Can you work these out from the model? Positions are in its coordinate system, mm. Round coordinates to 2 decimals unless told otherwise and drop trailing zeros. Order: outer loops, then holes, each group sorted by start corner. A loop starts at its lowest first (then second) coordinate and runs counter-clockwise, first axis right, second up. Notation, with made-up numbers: M 43,46.5 L 76,46.5 A38 ccw 76,85.5 Z; hole C 44,64.25 d3. An arc over 180 degrees is marked long. Answer as a JSON object with one key per item and string values. Group by question number.
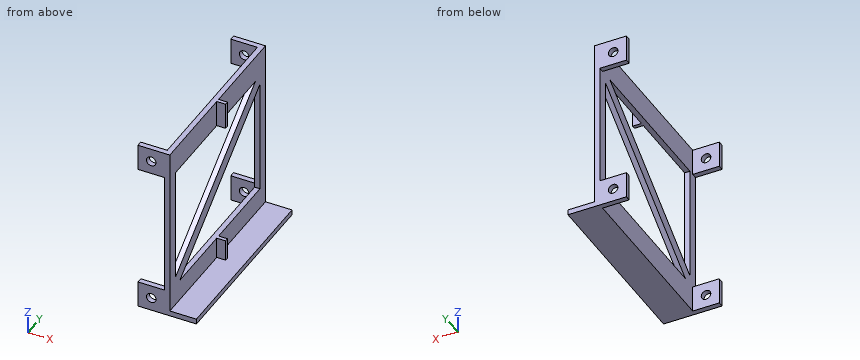
```python
from build123d import *

# Parameters (mm, degrees)
SKETCH2_W           = 15
SKETCH2_H           = 15
BOSS_EXTRUDE1_DEPTH = 3
SKETCH3_W           = 3
SKETCH3_H           = 15
BOSS_EXTRUDE2_DEPTH = 104
SKETCH4_W           = 15
SKETCH4_H           = 3
BOSS_EXTRUDE3_DEPTH = 15
SKETCH5_R           = 2.7
CUT_EXTRUDE1_DEPTH  = 105.999550604
SKETCH6_W           = 15
SKETCH6_H           = 2
BOSS_EXTRUDE4_DEPTH = 5
BOSS_EXTRUDE5_DEPTH = 3
SKETCH9_W           = 3
SKETCH9_H           = 104
BOSS_EXTRUDE6_DEPTH = 15


with BuildPart() as part:
    # Sketch2 → Boss-Extrude1 (new body)
    with BuildSketch(Plane(origin=(0, 0, 0), x_dir=(1, 0, 0), z_dir=(0, 1, 0))):
        with Locations((-4.400493642, 0.702675063)):
            Rectangle(SKETCH2_W, SKETCH2_H)
    extrude(amount=BOSS_EXTRUDE1_DEPTH)

    # Sketch3 → Boss-Extrude2 (add)
    with BuildSketch(Plane(origin=(0, 0, 0), x_dir=(1, 0, 0), z_dir=(0, 1, 0))):
        with Locations((4.599506358, 0.702675063)):
            Rectangle(SKETCH3_W, SKETCH3_H)
    extrude(amount=BOSS_EXTRUDE2_DEPTH)

    # Sketch4 → Boss-Extrude3 (add)
    with BuildSketch(Plane.ZY.offset(-3.099506358)):
        with Locations((-0.702675063, 102.5)):
            Rectangle(SKETCH4_W, SKETCH4_H)
    extrude(amount=BOSS_EXTRUDE3_DEPTH)

    # Sketch5 → Cut-Extrude1 (cut, through all)
    with BuildSketch(Plane.XZ):
        with Locations(Location((-4.400493642, -0.702675063, 0), (0, 0, 270))):
            Circle(SKETCH5_R)
    extrude(amount=-CUT_EXTRUDE1_DEPTH, mode=Mode.SUBTRACT)

    # Sketch6 → Boss-Extrude4 (add)
    with BuildSketch(Plane(origin=(6.099506358, 0, 0), x_dir=(0, 0, -1), z_dir=(1, 0, 0))):
        with Locations((0.702675063, 52)):
            Rectangle(SKETCH6_W, SKETCH6_H)
    extrude(amount=BOSS_EXTRUDE4_DEPTH)


with BuildPart() as body_2:
    # Body-Move/Copy2: copy of part
    add(part.part.moved(Location((0, 0, 85))))


with BuildPart() as part_1:
    add(part.part)

    add(body_2.part)  # Boss-Extrude5 merges body 2
    # Sketch8 → Boss-Extrude5 (add)
    with BuildSketch(Plane.ZY.offset(-6.099506358)):
        Polygon((6.797324937, 104), (76.797324937, 104), (76.797324937, 98), (76.797324937, 93), (11.797324937, 6), (76.797324937, 6), (76.797324937, 0), (6.797324937, 0), (6.797324937, 6), (6.797324937, 11), (71.797324937, 98), (6.797324937, 98), align=None)
    extrude(amount=BOSS_EXTRUDE5_DEPTH)

    # Sketch9 → Boss-Extrude6 (add)
    with BuildSketch(Plane(origin=(6.099506358, 0, 0), x_dir=(0, 0, -1), z_dir=(1, 0, 0))):
        with Locations((6.702675063, 52)):
            Rectangle(SKETCH9_W, SKETCH9_H)
    extrude(amount=BOSS_EXTRUDE6_DEPTH)


solid = part_1.part
```
1) If we section it at A-A on x = 1.5: Write out the boundary of the cut face in (y, z), plus the area to 3 significant figures.
2) If we section it at D-D on z = 19: Write out the boundary of the cut face in (x, y).
3) If we section it at B-B on y = 14: Write out the boundary of the cut face in (x, z).
4) I need wall thicknesses on line 1 along Y through (x, z) = (-10, 85); line 2 along Y through (x, z) = (6, 71.5); line 3 along Y through (x, z) = (8, 87.5). Which ranges of each line are inside material? Lowest first, please.
5) For pin 1 (10 mm diameter, centred on y = 10.5, z = 54, fed in from +X); pin 2 (2 mm diameter, centred on x = 7.5, z = 4.5, fed in from +Y); pin 3 (12 mm diameter, centred on x = -6, z = 1, fed in from -Y); pin 4 (4.5 mm diameter, centred on x = 17, y = 52, fed in from +Z), each with a flat end and sliding along its axis, tell me the tip position at first contact or that it passes through.
6) If we section it at C-C on z = 5.5: Write out the boundary of the cut face in (x, y).
Findings:
{
 "1": {"outline": "M 0,-8.2 L 3,-8.2 L 3,6.8 L 0,6.8 Z; M 0,76.8 L 3,76.8 L 3,91.8 L 0,91.8 Z; M 101,-8.2 L 104,-8.2 L 104,6.8 L 101,6.8 Z; M 101,76.8 L 104,76.8 L 104,91.8 L 101,91.8 Z", "area": "180 mm^2"},
 "2": {"outline": "M 3.1,0 L 6.1,0 L 6.1,6 L 3.1,6 Z; M 3.1,15.64 L 6.1,15.64 L 6.1,27.33 L 3.1,27.33 Z; M 3.1,98 L 6.1,98 L 6.1,104 L 3.1,104 Z"},
 "3": {"outline": "M 3.1,-8.2 L 21.1,-8.2 L 21.1,-5.2 L 6.1,-5.2 L 6.1,6.8 L 3.1,6.8 Z; M 3.1,9.04 L 6.1,9.04 L 6.1,17.77 L 3.1,17.77 Z; M 3.1,76.8 L 6.1,76.8 L 6.1,91.8 L 3.1,91.8 Z"},
 "4": {"line 1": "y = 0 to 3, 101 to 104", "line 2": "y = 0 to 6, 85.91 to 97.6, 98 to 104", "line 3": "y = 51 to 53"},
 "5": {"pin 1": "stops at x = 6.1", "pin 2": "stops at y = 53", "pin 3": "stops at y = 0", "pin 4": "stops at z = -5.2"},
 "6": {"outline": "M -11.9,0 L 6.1,0 L 6.1,51 L 11.1,51 L 11.1,53 L 6.1,53 L 6.1,104 L -11.9,104 L -11.9,101 L 3.1,101 L 3.1,3 L -11.9,3 Z"}
}
